The listing builds one solid part. Answer for the finished solid, in the listing's coordinates (mm). Give positions to 0.01 mm unless a question says otherwise; leave off trailing zeros. Answer in a Markdown table with one row per item.
from build123d import *

# Parameters (mm, degrees)
ESQUISSE1_W                          = 250
ESQUISSE1_H                          = 500
BOSS_EXTRU_1_DEPTH                   = 3
ENL_V_MAT_EXTRU_1_REACH              = 561.025
ESQUISSE2_R                          = 5
R_P_TITION_LIN_AIRE1_COUNT           = 2
R_P_TITION_LIN_AIRE1_PITCH           = 225
R_P_TITION_LIN_AIRE2_COUNT           = 2
R_P_TITION_LIN_AIRE2_PITCH           = 470
R_P_TITION_LIN_AIRE2_COPY_1_REACH    = 561.025
R_P_TITION_LIN_AIRE2_COPY_1_SKETCH_R = 5


with BuildPart() as part:
    # Esquisse1 → Boss.-Extru.1 (new body)
    with BuildSketch(Plane.XY):
        with Locations((125, 250)):
            Rectangle(ESQUISSE1_W, ESQUISSE1_H)
    extrude(amount=BOSS_EXTRU_1_DEPTH)

    # Esquisse2 → Enlèv. mat.-Extru.1 (cut, up to next)
    with BuildSketch(Plane.XY.offset(3), mode=Mode.PRIVATE) as enl_v_mat_extru_1_sk1:
        with Locations((12.561884872, 11.993805772)):
            Circle(ESQUISSE2_R)
    enl_v_mat_extru_1_tool1 = extrude(enl_v_mat_extru_1_sk1.sketch, amount=-ENL_V_MAT_EXTRU_1_REACH, mode=Mode.PRIVATE) & part.part
    enl_v_mat_extru_1 = enl_v_mat_extru_1_tool1.solids().sort_by_distance((12.561885, 11.993806, 3))[0]
    add(enl_v_mat_extru_1, mode=Mode.SUBTRACT)

    # Répétition linéaire1: Enlèv. mat.-Extru.1 ×2
    with Locations(*[(i * R_P_TITION_LIN_AIRE1_PITCH, 0, 0) for i in range(1, R_P_TITION_LIN_AIRE1_COUNT)]):
        add(enl_v_mat_extru_1, mode=Mode.SUBTRACT)

    # Répétition linéaire2: Enlèv. mat.-Extru.1 ×2
    with Locations(*[(0, i * R_P_TITION_LIN_AIRE2_PITCH, 0) for i in range(1, R_P_TITION_LIN_AIRE2_COUNT)]):
        add(enl_v_mat_extru_1, mode=Mode.SUBTRACT)

    # Répétition linéaire2 copy 1 sketch → Répétition linéaire2 copy 1 (cut, up to next)
    with BuildSketch(Plane(origin=(225, 470, 3), x_dir=(1, 0, 0), z_dir=(0, 0, 1)), mode=Mode.PRIVATE) as r_p_tition_lin_aire2_copy_1_sk1:
        with Locations((12.561884872, 11.993805772)):
            Circle(R_P_TITION_LIN_AIRE2_COPY_1_SKETCH_R)
    r_p_tition_lin_aire2_copy_1_tool1 = extrude(r_p_tition_lin_aire2_copy_1_sk1.sketch, amount=-R_P_TITION_LIN_AIRE2_COPY_1_REACH, mode=Mode.PRIVATE) & part.part
    add(r_p_tition_lin_aire2_copy_1_tool1.solids().sort_by_distance((237.561885, 481.993806, 3))[0], mode=Mode.SUBTRACT)


solid = part.part
Item 1: Consider line 1 (Y direction, x = 233.5, z = 0.6); line 2 (Y direction, x = 236, z = 0.7). Determine where each line is inside the solid, lowest interval first.
Answer block:
| item | result |
|---|---|
| line 1 | 0 to 9.08, 14.91 to 479.08, 484.91 to 500 |
| line 2 | 0 to 7.24, 16.74 to 477.24, 486.74 to 500 |
Item 2: Determine the mould class of faces 1 (the face through (123, 254, 0)), 2 (the face through (236.91, 486.95, 1.52)) for opening direction Y: pulls with the +Y half, pulls with the -Y half, needs draft (parallel to the pull), parting line crosses it, or undercut.
Answer block:
| item | result |
|---|---|
| face 1 | needs draft |
| face 2 | undercut |
Item 3: This flat-tipped pin is pushed along its axis until it touches: P1, Ø6, axis at x = 12.56, y = 481.99, coming from the -Z side. Where does it stop, or does it pass through?
Answer block:
| item | result |
|---|---|
| P1 | through |
